The listing builds one solid part. Answer for the finished solid, in the listing's coordinates (mm). A direction names the side the tool comes from. Round coordinates to 2 decimals unless told otherwise and drop trailing zeros. Order: outer loops, then holes, each group sorted by start corner. A loop starts at its lowest first (then second) coordinate and runs counter-clockwise, first axis right, second up. Notation, with made-up numbers: (27.25, 38) - (66.25, 38) arc R28 cw to (66.25, 66) - close; hole circle Ø2 at (59.5, 11.25). An arc over 180 degrees is marked (long way). Use CSV: the item, a comma, the result in double quotes. Start each with the question number.
Item 1: Determine the mould class of faces 1 (the flat face through (-15, -0.3, -1.6)), 2 (the cylindrical face through (9.53, 17.9, -2.86)), 3 (the flat face through (0, -25, -3)), 4 (the flat face through (0, 25, -3)) for opening direction Y: +Y half, -Y half, draft (parallel to the pull), parting line (faces both ways), or undercut.
Item 2: Find section A-A, the plane z = -2.8. Give the vertices of the cut face in (x, y).
Item 3: Find section D-D, the plane x = 0. Give the vertices of the cut face in (y, z), plus the area to 3 significant figures.
Item 4: For faces 5 (the flat face through (9, 17.25, -5)), 6 (the cylindrical face through (9.53, -22.1, -2.86)), determine the directions among +Z, -Z, +X, -X, +Y, -Y from which every point of the face is accessible in a straight line to the end or side of a thin tool.
Item 5: Find section C-C, the plane x = 9. Give the vertices of the cut face in (y, z), plus the area to 3 significant figures.
Item 6: Straight lines are drawn through the part: line 1 along Y through (x, z) = (13.5, -4.25); line 2 along Y through (x, z) = (-11.25, -3.2); line 3 along Y through (x, z) = (-6, -2.4). For each, find the intervals that lie inside material, in ascending order. Write a range as [from, to].
Item 7: Find section B-B, the plane y = 0. Give the vertices of the cut face in (x, z), plus the area to 3 significant figures.
Item 8: Flat-ended cylindrical pins translate along their axes: P1, Ø6, axis at x = -9.5, y = 2, coming from the -Z side; P2, Ø2, axis at x = 5, y = 16, coming from the -Z side. Find the tip coordinate at first contact, or state that the pin passes through.
```python
from build123d import *

# Parameters (mm, degrees)
PAD_DEPTH       = 15
PAD_DEPTH_BACK  = 15
SKETCH001_R     = 2.15
HOLE_DEPTH      = 25
SKETCH003_R     = 4.8
POCKET001_DEPTH = 5


with BuildPart() as part:
    # Sketch → Pad (new body, two sides)
    with BuildSketch(Plane.YZ) as pad_sk:
        Polygon((-25, 0), (-25, -5.8), (-17.25, -5.8), (-17.25, -3.3), (-15.25, -3.3), (-15.25, -1.8), (15.25, -1.8), (15.25, -3.3), (17.25, -3.3), (17.25, -5.8), (25, -5.8), (25, 0), align=None)
    extrude(amount=PAD_DEPTH)
    extrude(pad_sk.sketch, amount=-PAD_DEPTH_BACK)

    # Sketch001 → Hole (cut)
    with BuildSketch(Plane.XY):
        with Locations((-10, 20)):
            Circle(SKETCH001_R)
        with Locations((0, 17.5)):
            Circle(SKETCH001_R)
        with Locations((10, 20)):
            Circle(SKETCH001_R)
        with Locations((10, -20)):
            Circle(SKETCH001_R)
        with Locations((0, -17.5)):
            Circle(SKETCH001_R)
        with Locations((-10, -20)):
            Circle(SKETCH001_R)
    extrude(amount=-HOLE_DEPTH, mode=Mode.SUBTRACT)

    # Sketch003 → Pocket001 (cut)
    with BuildSketch(Plane.XY):
        with Locations((-8, 0)):
            Circle(SKETCH003_R)
        with Locations((8, 0)):
            Circle(SKETCH003_R)
    extrude(amount=-POCKET001_DEPTH, mode=Mode.SUBTRACT)


solid = part.part
```
Worked out:
1,face 1,"draft"
1,face 2,"undercut"
1,face 3,"-Y half"
1,face 4,"+Y half"
2,outline,"(-15, -25) - (15, -25) - (15, -15.25) - (-15, -15.25) - close; (-15, 15.25) - (15, 15.25) - (15, 25) - (-15, 25) - close; hole circle Ø4.3 at (-10, -20); hole circle Ø4.3 at (-10, 20); hole circle Ø4.3 at (0, -17.5); hole circle Ø4.3 at (0, 17.5); hole circle Ø4.3 at (10, -20); hole circle Ø4.3 at (10, 20)"
3,outline,"(-25, -5.8) - (-19.65, -5.8) - (-19.65, 0) - (-25, 0) - close; (-15.35, -3.3) - (-15.25, -3.3) - (-15.25, -1.8) - (15.25, -1.8) - (15.25, -3.3) - (15.35, -3.3) - (15.35, 0) - (-15.35, 0) - close; (19.65, -5.8) - (25, -5.8) - (25, 0) - (19.65, 0) - close"
3,area,"118 mm²"
4,face 5,"-Z, +X, -X"
4,face 6,"+Z, -Z"
5,outline,"(-25, -5.8) - (-21.9, -5.8) - (-21.9, 0) - (-25, 0) - close; (-18.1, -5.8) - (-17.25, -5.8) - (-17.25, -3.3) - (-15.25, -3.3) - (-15.25, -1.8) - (-4.69, -1.8) - (-4.69, 0) - (-18.1, 0) - close; (4.69, -1.8) - (15.25, -1.8) - (15.25, -3.3) - (17.25, -3.3) - (17.25, -5.8) - (18.1, -5.8) - (18.1, 0) - (4.69, 0) - close; (21.9, -5.8) - (25, -5.8) - (25, 0) - (21.9, 0) - close"
5,area,"96.9 mm²"
6,line 1,"y = [-25, -17.25], [17.25, 25]"
6,line 2,"y = [-25, -21.75], [-18.25, -15.25], [15.25, 18.25], [21.75, 25]"
6,line 3,"y = [-25, -15.25], [15.25, 25]"
7,outline,"(-15, -1.8) - (-12.8, -1.8) - (-12.8, 0) - (-15, 0) - close; (-3.2, -1.8) - (3.2, -1.8) - (3.2, 0) - (-3.2, 0) - close; (12.8, -1.8) - (15, -1.8) - (15, 0) - (12.8, 0) - close"
7,area,"19.4 mm²"
8,P1,"stops at z = -1.8"
8,P2,"stops at z = -3.3"
